from build123d import *

# Parameters (mm, degrees)
F0_W     = 106.68
F0_H     = 106.68
F1_DEPTH = 88.9
F2_T     = -3.81
F3_W     = 101.6
F3_H     = 50.8
F4_DEPTH = 25.4


with BuildPart() as f1:
    # F0 (on Front) → F1 (new body)
    with BuildSketch(Plane.XZ):
        with Locations((53.34, 53.34)):
            Rectangle(F0_W, F0_H)
    extrude(amount=-F1_DEPTH)

    # F2
    f2_openings = [f1.faces().sort_by_distance(p)[0] for p in [
        (53.34, 0, 53.34),
    ]]
    offset(amount=F2_T, openings=f2_openings)

    # F3 (on face) → F4 (cut)
    with BuildSketch(Plane(origin=(0, 88.9, 0), x_dir=(-1, 0, 0), z_dir=(0, 1, 0))):
        with Locations((-53.34, 29.175188)):
            Rectangle(F3_W, F3_H)
    extrude(amount=-F4_DEPTH, mode=Mode.SUBTRACT)


solid = f1.part
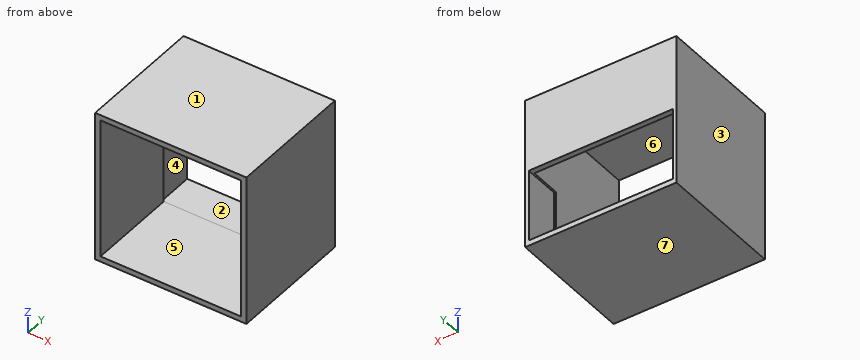
Input: part model. Units: mm. Frame: model coordinates. Face numbers are marked on the shaded views. A direction names the side the tool comes from. Coordinates: 2 decimals unless noted, no trailing zeros. Write each loop counter-clockwise with the first axis right and the second up, starting at its lowest first coordinate (ties: lowest second). Pieces come first, ordered by that corner, then holes. Notation, with made-up numbers: M -5.75,61.25 L 0.25,61.25 A19 ccw 0.25,72.25 Z; hole C -12.5,44.25 d1. An arc over 180 degrees is marked long. Answer as a JSON object with one key per item and string values. Group by question number.
(1) Section C-C on y = 11. Output: boundary loops of the cut face in (x, z), plus the area to 3 significant figures.
(2) Section A-A on z = 35.5. Output: boundary loops of the cut face in (x, y), plus the area to 3 significant figures.
(3) Section D-D on z = 72.5. Output: boundary loops of the cut face in (x, y), plus the area to 3 significant figures.
(4) Ray query, line 1 along X through (y, z) = (53.5, 71.5); line 2 along X through (y, z) = (75, 23.5). Return the intervals inside material, ascending. Write a range as [from, to].
(5) Set-up query: the marked faces 4, 5, 6 and 7. Return all of +Z, -Z, +X, -X, +Y, -Y with unobstructed straight access to the full face (end or side cutting, diameter ignored); none if empty.
(6) Contact query for a flat-ended pin moving along its axis: P1, Ø8, axis at x = 63.5, z = 72, coming from the -Y side. Output: stop coordinate, or through.
(7) Mould query, pull axis X, two halves, no side actions, for the marked faces 1, 2 and 3. Classes: pulls with the +X half, pulls with the -X half, needs draft (parallel to the pull), parting line crosses it, or undercut.
Result set:
{
 "1": {"outline": "M 0,0 L 106.68,0 L 106.68,106.68 L 0,106.68 Z; hole M 3.81,3.81 L 102.87,3.81 L 102.87,102.87 L 3.81,102.87 Z", "area": "1,570 mm2"},
 "2": {"outline": "M 0,0 L 3.81,0 L 3.81,63.5 L 2.54,63.5 L 2.54,88.9 L 0,88.9 Z; M 102.87,0 L 106.68,0 L 106.68,88.9 L 104.14,88.9 L 104.14,63.5 L 102.87,63.5 Z", "area": "613 mm2"},
 "3": {"outline": "M 0,0 L 3.81,0 L 3.81,85.09 L 102.87,85.09 L 102.87,0 L 106.68,0 L 106.68,88.9 L 0,88.9 Z", "area": "1,050 mm2"},
 "4": {"line 1": "x = [0, 3.81], [102.87, 106.68]", "line 2": "x = [0, 2.54], [104.14, 106.68]"},
 "5": {"face 4": "+Y", "face 5": "+Y, -Y", "face 6": "-Y", "face 7": "-Z, +X, -X, +Y, -Y"},
 "6": {"P1": "stops at y = 85.09"},
 "7": {"face 1": "needs draft", "face 2": "undercut", "face 3": "pulls with the -X half"}
}
